Geometry: final body of the model. Coordinates: model frame, mm. Coordinates: 2 decimals unless noted, no trailing zeros. Order: outer loops, then holes, each group sorted by start corner. A loop starts at its lowest first (then second) coordinate and runs counter-clockwise, first axis right, second up. Notation, with made-up numbers: M -31.75,42.25 L 12.25,42.25 A22 cw 12.25,50.25 Z; hole C 42.5,19 d2. An arc over 180 degrees is marked long. Use CSV: the item, a comma, the result in double quotes. Start each with the question number.
1. First-contact query: P1, Ø4, axis at y = -7, z = -7, coming from the +X side; P2, Ø2, axis at x = 5, z = -6, coming from the -Y side; P3, Ø2, axis at x = 8, z = -4.5, coming from the +Y side; P4, Ø8, axis at x = -4, y = -7.5, coming from the -Z side. Flat tips, straight axial feed; report the tip coordinate or a pass-through.
2. Pull-direction query (X, two-part tool) for faces 1 (the cylindrical face through (4.57, 7.167, -3.945)), 2 (the cylindrical face through (10, 3.2, -3.9)), 3 (the flat face through (-9, 0, 0)); classes: pulls with the +X half, pulls with the -X half, needs draft (parallel to the pull), parting line crosses it, or undercut.
3. Section query D-D on y = 9. Return the cut outline in (x, z), and give its area (3 significant figures).
4. Section query C-C on z = -4.5. Return the cut outline in (x, y), and give its area (3 significant figures).
5. Section query A-A on x = 0. Return the cut outline in (y, z), and give its area (3 significant figures).
6. Material intervals for line 1 (Y direction, x = 0, z = -6); line 2 (X direction, y = 1.75, z = -3); line 3 (X direction, y = -6.5, z = -4.25), sorted ascending.
from build123d import *

# Parameters (mm, degrees)
SKETCH2_R           = 10.5
BOSS_EXTRUDE1_DEPTH = 8
SKETCH3_R           = 8.5
CUT_EXTRUDE1_DEPTH  = 9
CHAMFER1_SIZE       = 0.05
CHAMFER2_SIZE       = 0.05


with BuildPart() as part:
    # Sketch2 → Boss-Extrude1 (new body)
    with BuildSketch(Plane.XY):
        Circle(SKETCH2_R)
    extrude(amount=-BOSS_EXTRUDE1_DEPTH)

    # Sketch3 → Cut-Extrude1 (cut, through all)
    with BuildSketch(Plane.XY):
        Circle(SKETCH3_R)
    extrude(amount=-CUT_EXTRUDE1_DEPTH, mode=Mode.SUBTRACT)

    # Chamfer1
    chamfer1_edges = [part.edges().sort_by_distance(p)[0] for p in [
        (-8.5, 0, 0),
    ]]
    chamfer(chamfer1_edges, length=CHAMFER1_SIZE)

    # Chamfer2
    chamfer2_edges = [part.edges().sort_by_distance(p)[0] for p in [
        (-8.5, 0, -8),
    ]]
    chamfer(chamfer2_edges, length=CHAMFER2_SIZE)


solid = part.part
Results list:
1,P1,"stops at x = 9.23"
1,P2,"stops at y = -9.71"
1,P3,"stops at y = 7.83"
1,P4,"stops at z = -8"
2,face 1,"undercut"
2,face 2,"parting line crosses it"
2,face 3,"needs draft"
3,outline,"M -5.41,-8 L 5.41,-8 L 5.41,0 L -5.41,0 Z"
3,area,"86.5 mm²"
4,outline,"C 0,0 d21; hole C 0,0 d17"
4,area,"119 mm²"
5,outline,"M -10.5,-8 L -8.55,-8 L -8.5,-7.95 L -8.5,-0.05 L -8.55,0 L -10.5,0 Z; M 8.5,-7.95 L 8.55,-8 L 10.5,-8 L 10.5,0 L 8.55,0 L 8.5,-0.05 Z"
5,area,"32.0 mm²"
6,line 1,"y = -10.5 to -8.5, 8.5 to 10.5"
6,line 2,"x = -10.35 to -8.32, 8.32 to 10.35"
6,line 3,"x = -8.25 to -5.48, 5.48 to 8.25"
